Model file for the job. Use its own axes, mm. Face numbers are marked on the shaded views. A direction names the side the tool comes from. Coordinates: 2 decimals unless noted, no trailing zeros. Loops run counter-clockwise (first coordinate to the right, second up) from the corner with the lowest first, then second, coordinate; pieces in that order, holes last. Notation, with made-up numbers: (-6, 4) -> (49, 4) arc R34 cw to (49, 35) -> close; hole circle Ø9 at (39, 31). An arc over 180 degrees is marked (long way). Use one line per item in the form item = value.
```python
from build123d import *

# Parameters (mm, degrees)
F0_W      = 15
F0_H      = 30
F0_W_2    = 8
F0_H_2    = 2
F1_DEPTH  = 2
F2_DEPTH  = 38
F4_W      = 8
F4_H      = 19
F5_DEPTH  = 25
F6_D      = 4
F6_DEPTH  = 50
F6_TIP    = 1.2017212381
F7_R      = 2.5
F8_R      = 8
F10_DEPTH = 25


with BuildPart() as f1:
    # F0 (on Front) → F1 (new body)
    with BuildSketch(Plane.XZ):
        Polygon((9.5, -15), (9.5, 17), (-9.5, 17), (-9.5, -15), (-9.5, -17), (9.5, -17), align=None)
        Rectangle(F0_W, F0_H, mode=Mode.SUBTRACT)
        with Locations((13.5, -16)):
            Rectangle(F0_W_2, F0_H_2)
        with Locations((-13.5, -16)):
            Rectangle(F0_W_2, F0_H_2)
        Rectangle(F0_W, F0_H)
        with BuildLine():
            ThreePointArc((3.3443871458, 4.9814731375), (5.2946351562, 2.8225588679), (6, 0))
            ThreePointArc((6, 0), (-2.8225588679, -5.2946351562), (-3.3443871458, 4.9814731375))
            ThreePointArc((-3.3443871458, 4.9814731375), (0, 6), (3.3443871458, 4.9814731375))
        make_face(mode=Mode.SUBTRACT)
        with BuildLine():
            Line((-3.3443871458, 4.9814731375), (3.3443871458, 4.9814731375))
            ThreePointArc((3.3443871458, 4.9814731375), (0, 6), (-3.3443871458, 4.9814731375))
        make_face()
    extrude(amount=F1_DEPTH)

    # F0 (on Front) → F2 (join)
    with BuildSketch(Plane.XZ):
        Polygon((9.5, -15), (9.5, 17), (-9.5, 17), (-9.5, -15), (-9.5, -17), (9.5, -17), align=None)
        Rectangle(F0_W, F0_H, mode=Mode.SUBTRACT)
        with Locations((13.5, -16)):
            Rectangle(F0_W_2, F0_H_2)
        with Locations((-13.5, -16)):
            Rectangle(F0_W_2, F0_H_2)
    extrude(amount=-F2_DEPTH)

    # F4 (on offset) → F5 (cut)
    with BuildSketch(Plane.XY.offset(-15)):
        with Locations((-13.5, 28.5)):
            Rectangle(F4_W, F4_H)
        with Locations((13.5, 28.5)):
            Rectangle(F4_W, F4_H)
    extrude(amount=-F5_DEPTH, mode=Mode.SUBTRACT)

    # F6
    with Locations(Plane.XY.offset(-15)):
        with Locations((-13.5, 13), (13.5, 13)):
            Hole(F6_D / 2, depth=F6_DEPTH)
            with Locations((0, 0, -(F6_DEPTH + F6_TIP / 2))):  # 118° drill point
                Cone(0, F6_D / 2, F6_TIP, mode=Mode.SUBTRACT)

    # F7
    f7_edges = [f1.edges().sort_by_distance(p)[0] for p in [
        (9.5, -2, 1),
        (-9.5, -2, 1),
        (-9.5, 18, 17),
        (9.5, 18, 17),
        (0, -2, 17),
        (17.5, 19, -16),
        (-17.5, 19, -16),
    ]]
    fillet(f7_edges, radius=F7_R)

    # F8
    f8_edges = [f1.edges().sort_by_distance(p)[0] for p in [
        (-17.5, -2, -16),
        (17.5, -2, -16),
    ]]
    fillet(f8_edges, radius=F8_R)

    # F9 (on face) → F10 (cut)
    with BuildSketch(Plane(origin=(-9.5, 0, 0), x_dir=(0, -1, 0), z_dir=(-1, 0, 0))):
        Polygon((-19, -15), (-38, 14.5), (-38, -17), (-19, -17), align=None)
    extrude(amount=-F10_DEPTH, mode=Mode.SUBTRACT)


solid = f1.part
```
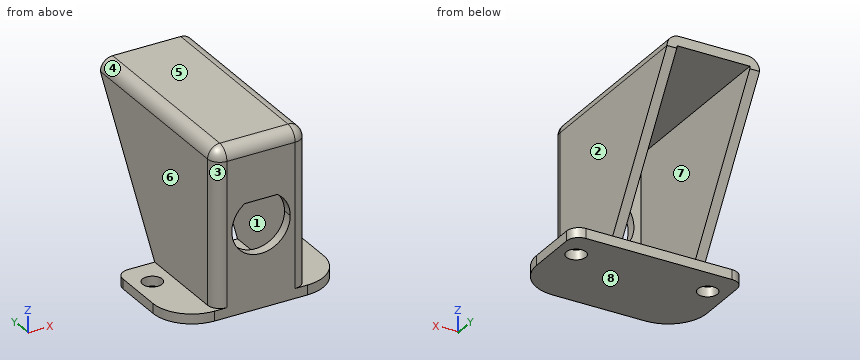
Q1. Wall check: line 1 along X through (y, z) = (10.5, 12); line 2 along Z through (x, y) = (-1.5, 6.5); line 3 along Y through (x, z) = (-3.5, -6.5). Give the ranges that are in metal, low to high.
Result:
line_1 = -9.5 to -7.5, 7.5 to 9.5
line_2 = -17 to -15, 15 to 17
line_3 = -2 to 0
Q2. Which spindle directions (+Z, -Z, +X, -X, +Y, -Y) get a long thin tool onto all of the face, cutting with end or side? Do the marked faces 1, 2, 3, 4 and 5. Say none if no direction does.
Result:
face_1 = +Y
face_2 = +Z, +X, +Y, -Y
face_3 = +Z, -X, -Y
face_4 = +Z, -X, +Y, -Y
face_5 = +Z, +X, -X, +Y, -Y
Q3. Mould opens along X. For the marked faces 6, 7 and 8 say: released by +X, released by -X, zero draft, split by the parting line, or undercut.
Result:
face_6 = released by -X
face_7 = undercut
face_8 = zero draft
Q4. Band-saw the part on D-D, the plane z = 11. Write the cut outline in (x, y).
Result:
outline = (-9.5, 0.5) arc R2.5 ccw to (-7, -2) -> (7, -2) arc R2.5 ccw to (9.5, 0.5) -> (9.5, 35.75) -> (7.5, 35.75) -> (7.5, 0) -> (-7.5, 0) -> (-7.5, 35.75) -> (-9.5, 35.75) -> close
Q5. Band-saw the part on B-B, the plane z = -1.5. Write the cut outline in (x, y), and give its area (3 significant figures).
Result:
outline = (-9.5, 0.5) arc R2.5 ccw to (-7, -2) -> (-5.81, -2) -> (-5.81, 0) -> (-7.5, 0) -> (-7.5, 27.69) -> (-9.5, 27.69) -> close; (5.81, -2) -> (7, -2) arc R2.5 ccw to (9.5, 0.5) -> (9.5, 27.69) -> (7.5, 27.69) -> (7.5, 0) -> (5.81, 0) -> close
area = 123 mm2
Q6. Band-saw the part on A-A, the plane x = 13. Write the cut outline in (y, z).
Result:
outline = (-1.19, -17) -> (11.06, -17) -> (11.06, -15) -> (-1.19, -15) -> close; (14.94, -17) -> (19, -17) -> (19, -15) -> (14.94, -15) -> close
Q7. Pin check, flat tips, straight feed: pin 1 Ø15 at (y, z) = (28, 6.5) entering from -X; pin 2 Ø5 at (y, z) = (25.5, 11.5) entering from +X; pin 3 Ø2 at (x, z) = (5.5, -16) entering from +Y; pin 4 Ø3 at (x, y) = (13.5, 13) entering from -Z. Stop position of each tip, or through.
Result:
pin_1 = -9.5
pin_2 = 9.5
pin_3 = 19
pin_4 = through
Q8. Band-saw the part on C-C, the plane y = 28.5. Write the cut outline in (x, z).
Result:
outline = (-9.5, -0.25) -> (-7.5, -0.25) -> (-7.5, 15) -> (7.5, 15) -> (7.5, -0.25) -> (9.5, -0.25) -> (9.5, 14.5) arc R2.5 ccw to (7, 17) -> (-7, 17) arc R2.5 ccw to (-9.5, 14.5) -> close
